Job drawing, mm, ordinate dimensions from the low corner. One solid piece. A direction names the side the tool comes from. Round coordinates to 2 decimals unless told otherwise and drop trailing zeros. Write each loop counter-clockwise with the first axis right and the second up, starting at its lowest first coordinate (ties: lowest second). Pieces come first, ordered by that corner, then holes. Notation, with made-up numbers: M 25.25,66.5 L 36.25,66.5 A20 cw 36.25,70.5 Z; hole C 86,68 d7. An arc over 180 degrees is marked long. Answer as a JSON object with one key per item and string values. Group by question number.
1. Band-saw the part on A-A, the plane z = 4. Write the cut outline in (x, y), plus the area to 3 significant figures.
2. Band-saw the part on C-C, the plane y = 4.5. Write the cut outline in (x, z).
3. Two-plate mould, pull along Y, no slides. Class the marked faces 4, 5, 6 and 7: +Y half, -Y half, draft (parallel to the pull), parting line (faces both ways), or undercut.
4. Drop flat-ended pins along their axis: pin 1 (1.7 mm diameter, centred on x = 1.5, y = 5, fed in from +Z); pin 2 (2 mm diameter, centred on x = 10.5, z = 2.5, fed in from -Y); pin 3 (2.5 mm diameter, centred on x = 6, z = 4, fed in from +Y). Give the stop position or say it passes through.
5. Drill centre lines: line 1 (X direction, y = 2.45, z = 4); line 2 (X direction, y = 4.5, z = 7.25); line 3 (X direction, y = 5.75, z = 3.25). Where is each one in solid material? Low to high. Write a range as from..to.
6. Band-saw the part on D-D, the plane z = 2. Write the cut outline in (x, y), plus the area to 3 significant figures.
7. Which spindle directions (+Z, -Z, +X, -X, +Y, -Y) get a long thin tool onto all of the face, cutting with end or side? Do the marked faces 1, 2 and 3. Say none if no direction does.
8. Band-saw the part on B-B, the plane x = 10.5. Write the cut outline in (y, z).
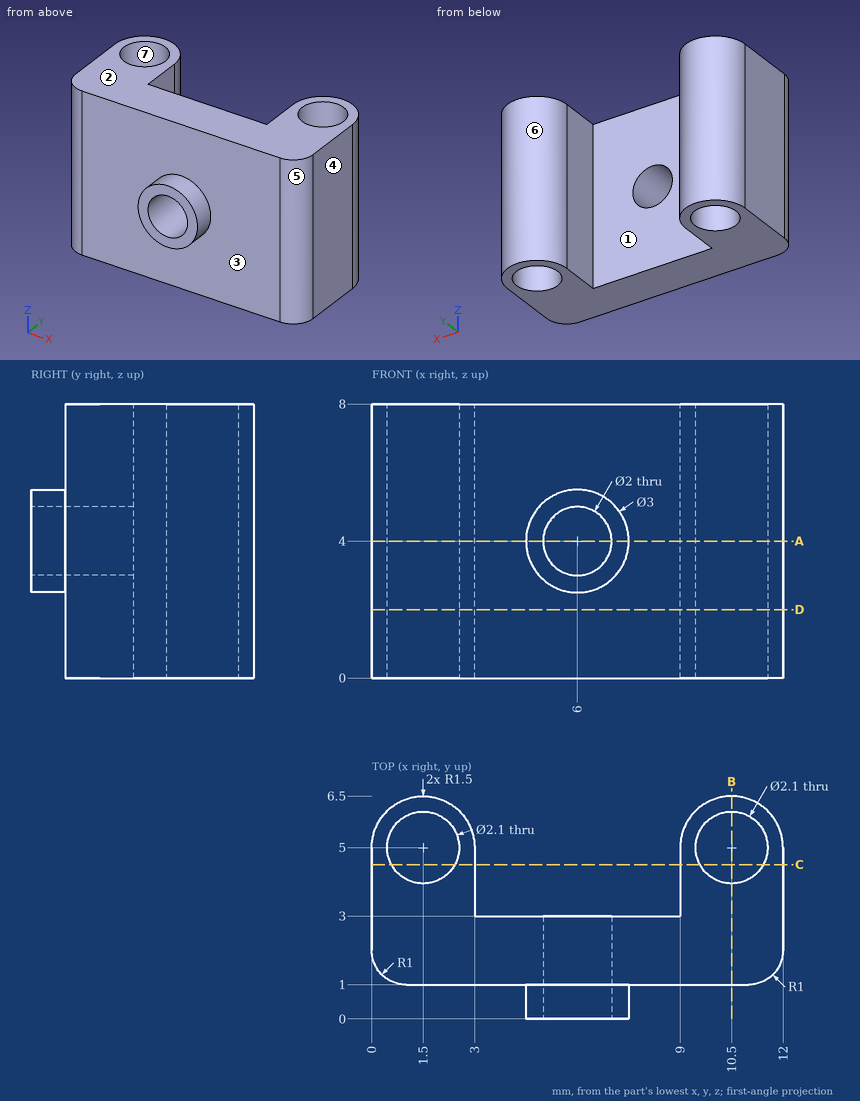
Worked answers:
{
 "1": {"outline": "M 0,2 A1 ccw 1,1 L 4.5,1 L 4.5,0 L 5,0 L 5,3 L 3,3 L 3,5 A1.5 ccw 0,5 Z; M 7,0 L 7.5,0 L 7.5,1 L 11,1 A1 ccw 12,2 L 12,5 A1.5 ccw 9,5 L 9,3 L 7,3 Z; hole C 1.5,5 d2.1; hole C 10.5,5 d2.1", "area": "32.7 mm^2"},
 "2": {"outline": "M 0,0 L 0.58,0 L 0.58,8 L 0,8 Z; M 2.42,0 L 3,0 L 3,8 L 2.42,8 Z; M 9,0 L 9.58,0 L 9.58,8 L 9,8 Z; M 11.42,0 L 12,0 L 12,8 L 11.42,8 Z"},
 "3": {"face 4": "draft", "face 5": "-Y half", "face 6": "+Y half", "face 7": "undercut"},
 "4": {"pin 1": "passes through", "pin 2": "stops at y = 1", "pin 3": "stops at y = 3"},
 "5": {"line 1": "x = 0..5, 7..12", "line 2": "x = 0..0.58, 2.42..3, 9..9.58, 11.42..12", "line 3": "x = 0.2..0.77, 2.23..2.8, 9.2..9.77, 11.23..11.8"},
 "6": {"outline": "M 0,2 A1 ccw 1,1 L 11,1 A1 ccw 12,2 L 12,5 A1.5 ccw 9,5 L 9,3 L 3,3 L 3,5 A1.5 ccw 0,5 Z; hole C 1.5,5 d2.1; hole C 10.5,5 d2.1", "area": "35.7 mm^2"},
 "7": {"face 1": "+Z, -Z, +Y", "face 2": "+Z, +X, -X, +Y, -Y", "face 3": "-Y"},
 "8": {"outline": "M 1,0 L 3.95,0 L 3.95,8 L 1,8 Z; M 6.05,0 L 6.5,0 L 6.5,8 L 6.05,8 Z"}
}
